Model file for the job. Use its own axes, mm. A direction names the side the tool comes from. Give positions to 0.01 mm unless a question says otherwise; leave off trailing zeros. Write each loop counter-clockwise with the first axis right and the second up, starting at its lowest first coordinate (ties: lowest second). Pieces come first, ordered by that corner, then holes. Notation, with made-up numbers: (-10.5, 86) - (35.5, 86) arc R5 cw to (35.5, 91) - close; hole circle Ø9 at (75.25, 42.5). An arc over 180 degrees is marked (long way). Use CSV: the item, a comma, the result in double quotes.
from build123d import *

# Parameters (mm, degrees)
SKETCH1_W           = 609.6
SKETCH1_H           = 304.8
SKETCH1_W_2         = 93
SKETCH1_H_2         = 93
BOSS_EXTRUDE1_DEPTH = 15.24
SKETCH2_W           = 609.6
SKETCH2_H           = 304.8
BOSS_EXTRUDE2_DEPTH = 3.175
SKETCH3_W           = 609.6
SKETCH3_H           = 304.8
SKETCH3_W_2         = 603.25
SKETCH3_H_2         = 254
BOSS_EXTRUDE3_DEPTH = 30.48
SKETCH4_OUTSIDE_W   = 748.262
SKETCH4_OUTSIDE_H   = 443.462
SKETCH4_OUTSIDE_W_2 = 609.6
SKETCH4_OUTSIDE_H_2 = 260.35
CUT_EXTRUDE1_DEPTH  = 45.72
SKETCH5_R           = 3.4925
CUT_EXTRUDE2_DEPTH  = 344.830071983
SKETCH6_W           = 327.140785269
SKETCH6_H           = 256.091806272
TEMPORARY_CUT_DEPTH = 430.914472374
SKETCH7_W           = 260.35
SKETCH7_H           = 48.895
BOSS_EXTRUDE4_DEPTH = 3.175


with BuildPart() as part:
    # Sketch1 → Boss-Extrude1 (new body)
    with BuildSketch(Plane(origin=(0, 0, 0), x_dir=(1, 0, 0), z_dir=(0, 1, 0))):
        Rectangle(SKETCH1_W, SKETCH1_H)
        with Locations((-48.0875, 29.7)):
            Rectangle(SKETCH1_W_2, SKETCH1_H_2, mode=Mode.SUBTRACT)
        with Locations((-144.2625, 29.7)):
            Rectangle(SKETCH1_W_2, SKETCH1_H_2, mode=Mode.SUBTRACT)
        with Locations((-144.2625, -66.475)):
            Rectangle(SKETCH1_W_2, SKETCH1_H_2, mode=Mode.SUBTRACT)
        with Locations((-48.0875, -66.475)):
            Rectangle(SKETCH1_W_2, SKETCH1_H_2, mode=Mode.SUBTRACT)
        with Locations((-240.4375, 29.7)):
            Rectangle(SKETCH1_W_2, SKETCH1_H_2, mode=Mode.SUBTRACT)
        with Locations((-240.4375, -66.475)):
            Rectangle(SKETCH1_W_2, SKETCH1_H_2, mode=Mode.SUBTRACT)
        with Locations((48.0875, 29.7)):
            Rectangle(SKETCH1_W_2, SKETCH1_H_2, mode=Mode.SUBTRACT)
        with Locations((48.0875, -66.475)):
            Rectangle(SKETCH1_W_2, SKETCH1_H_2, mode=Mode.SUBTRACT)
        with Locations((144.2625, 29.7)):
            Rectangle(SKETCH1_W_2, SKETCH1_H_2, mode=Mode.SUBTRACT)
        with Locations((144.2625, -66.475)):
            Rectangle(SKETCH1_W_2, SKETCH1_H_2, mode=Mode.SUBTRACT)
        with Locations((240.4375, 29.7)):
            Rectangle(SKETCH1_W_2, SKETCH1_H_2, mode=Mode.SUBTRACT)
        with Locations((240.4375, -66.475)):
            Rectangle(SKETCH1_W_2, SKETCH1_H_2, mode=Mode.SUBTRACT)
    extrude(amount=BOSS_EXTRUDE1_DEPTH)

    # Sketch2 → Boss-Extrude2 (add)
    with BuildSketch(Plane(origin=(0, 0, 0), x_dir=(-1, 0, 0), z_dir=(0, -1, 0))):
        Rectangle(SKETCH2_W, SKETCH2_H)
    extrude(amount=BOSS_EXTRUDE2_DEPTH)

    # Sketch3 → Boss-Extrude3 (add)
    with BuildSketch(Plane(origin=(0, 15.24, 0), x_dir=(1, 0, 0), z_dir=(0, 1, 0))):
        Rectangle(SKETCH3_W, SKETCH3_H)
        Rectangle(SKETCH3_W_2, SKETCH3_H_2, mode=Mode.SUBTRACT)
    extrude(amount=BOSS_EXTRUDE3_DEPTH)

    # Sketch4 outside → Cut-Extrude1 (cut)
    with BuildSketch(Plane(origin=(0, 45.72, 0), x_dir=(1, 0, 0), z_dir=(0, 1, 0))):
        Rectangle(SKETCH4_OUTSIDE_W, SKETCH4_OUTSIDE_H)
        Rectangle(SKETCH4_OUTSIDE_W_2, SKETCH4_OUTSIDE_H_2, mode=Mode.SUBTRACT)
    extrude(amount=-CUT_EXTRUDE1_DEPTH, mode=Mode.SUBTRACT)

    # Sketch5 → Cut-Extrude2 (cut, through all)
    with BuildSketch(Plane(origin=(0, 0, 0), x_dir=(1, 0, 0), z_dir=(0, 1, 0))):
        with Locations(Location((-292.1, -139.7, 0), (0, 0, 270))):
            Circle(SKETCH5_R)
        with Locations(Location((-266.7, -139.7, 0), (0, 0, 270))):
            Circle(SKETCH5_R)
        with Locations(Location((-241.3, -139.7, 0), (0, 0, 270))):
            Circle(SKETCH5_R)
        with Locations(Location((-215.9, -139.7, 0), (0, 0, 270))):
            Circle(SKETCH5_R)
        with Locations(Location((-190.5, -139.7, 0), (0, 0, 270))):
            Circle(SKETCH5_R)
        with Locations(Location((-165.1, -139.7, 0), (0, 0, 270))):
            Circle(SKETCH5_R)
        with Locations(Location((-139.7, -139.7, 0), (0, 0, 270))):
            Circle(SKETCH5_R)
        with Locations(Location((-114.3, -139.7, 0), (0, 0, 270))):
            Circle(SKETCH5_R)
        with Locations(Location((-88.9, -139.7, 0), (0, 0, 270))):
            Circle(SKETCH5_R)
        with Locations(Location((-63.5, -139.7, 0), (0, 0, 270))):
            Circle(SKETCH5_R)
        with Locations(Location((-38.1, -139.7, 0), (0, 0, 270))):
            Circle(SKETCH5_R)
        with Locations(Location((-12.7, -139.7, 0), (0, 0, 270))):
            Circle(SKETCH5_R)
        with Locations(Location((12.7, 139.7, 0), (0, 0, 270))):
            Circle(SKETCH5_R)
        with Locations(Location((38.1, 139.7, 0), (0, 0, 270))):
            Circle(SKETCH5_R)
        with Locations(Location((63.5, 139.7, 0), (0, 0, 270))):
            Circle(SKETCH5_R)
        with Locations(Location((88.9, 139.7, 0), (0, 0, 270))):
            Circle(SKETCH5_R)
        with Locations(Location((114.3, 139.7, 0), (0, 0, 270))):
            Circle(SKETCH5_R)
        with Locations(Location((139.7, 139.7, 0), (0, 0, 270))):
            Circle(SKETCH5_R)
        with Locations(Location((165.1, 139.7, 0), (0, 0, 270))):
            Circle(SKETCH5_R)
        with Locations(Location((190.5, 139.7, 0), (0, 0, 270))):
            Circle(SKETCH5_R)
        with Locations(Location((215.9, 139.7, 0), (0, 0, 270))):
            Circle(SKETCH5_R)
        with Locations(Location((241.3, 139.7, 0), (0, 0, 270))):
            Circle(SKETCH5_R)
        with Locations(Location((-292.1, 139.7, 0), (0, 0, 270))):
            Circle(SKETCH5_R)
        with Locations(Location((-266.7, 139.7, 0), (0, 0, 270))):
            Circle(SKETCH5_R)
        with Locations(Location((-241.3, 139.7, 0), (0, 0, 270))):
            Circle(SKETCH5_R)
        with Locations(Location((-215.9, 139.7, 0), (0, 0, 270))):
            Circle(SKETCH5_R)
        with Locations(Location((-190.5, 139.7, 0), (0, 0, 270))):
            Circle(SKETCH5_R)
        with Locations(Location((-165.1, 139.7, 0), (0, 0, 270))):
            Circle(SKETCH5_R)
        with Locations(Location((-139.7, 139.7, 0), (0, 0, 270))):
            Circle(SKETCH5_R)
        with Locations(Location((-114.3, 139.7, 0), (0, 0, 270))):
            Circle(SKETCH5_R)
        with Locations(Location((-88.9, 139.7, 0), (0, 0, 270))):
            Circle(SKETCH5_R)
        with Locations(Location((-63.5, 139.7, 0), (0, 0, 270))):
            Circle(SKETCH5_R)
        with Locations(Location((-38.1, 139.7, 0), (0, 0, 270))):
            Circle(SKETCH5_R)
        with Locations(Location((-12.7, 139.7, 0), (0, 0, 270))):
            Circle(SKETCH5_R)
        with Locations(Location((266.7, 139.7, 0), (0, 0, 270))):
            Circle(SKETCH5_R)
        with Locations(Location((292.1, 139.7, 0), (0, 0, 270))):
            Circle(SKETCH5_R)
        with Locations(Location((12.7, -139.7, 0), (0, 0, 270))):
            Circle(SKETCH5_R)
        with Locations(Location((38.1, -139.7, 0), (0, 0, 270))):
            Circle(SKETCH5_R)
        with Locations(Location((63.5, -139.7, 0), (0, 0, 270))):
            Circle(SKETCH5_R)
        with Locations(Location((88.9, -139.7, 0), (0, 0, 270))):
            Circle(SKETCH5_R)
        with Locations(Location((114.3, -139.7, 0), (0, 0, 270))):
            Circle(SKETCH5_R)
        with Locations(Location((139.7, -139.7, 0), (0, 0, 270))):
            Circle(SKETCH5_R)
        with Locations(Location((165.1, -139.7, 0), (0, 0, 270))):
            Circle(SKETCH5_R)
        with Locations(Location((190.5, -139.7, 0), (0, 0, 270))):
            Circle(SKETCH5_R)
        with Locations(Location((215.9, -139.7, 0), (0, 0, 270))):
            Circle(SKETCH5_R)
        with Locations(Location((241.3, -139.7, 0), (0, 0, 270))):
            Circle(SKETCH5_R)
        with Locations(Location((266.7, -139.7, 0), (0, 0, 270))):
            Circle(SKETCH5_R)
        with Locations(Location((292.1, -139.7, 0), (0, 0, 270))):
            Circle(SKETCH5_R)
    extrude(amount=-CUT_EXTRUDE2_DEPTH, mode=Mode.SUBTRACT)

    # Sketch6 → Temporary_Cut (cut, through all)
    with BuildSketch(Plane(origin=(-94.5875, 0, 0), x_dir=(0, 0, -1), z_dir=(1, 0, 0))):
        with Locations((-7.828616148, 44.910513642)):
            Rectangle(SKETCH6_W, SKETCH6_H)
    extrude(amount=TEMPORARY_CUT_DEPTH, mode=Mode.SUBTRACT)

    # Sketch7 → Boss-Extrude4 (add)
    with BuildSketch(Plane(origin=(-94.5875, 0, 0), x_dir=(0, 0, -1), z_dir=(1, 0, 0))):
        with Locations((0, 21.2725)):
            Rectangle(SKETCH7_W, SKETCH7_H)
    extrude(amount=BOSS_EXTRUDE4_DEPTH)


solid = part.part
(1) Wall check: probe 1 along Z at (x, y) = (-210, 10) (3 decimals); probe 2 along Z at (x, y) = (-190.5, -0.9); probe 3 along Z at (x, y) = (-279, 41) (3 decimals). Give the ranges that are in metal, low to high. Write a range as [from, to].
Checked values:
probe 1,"z = [-130.175, -76.2], [16.8, 19.975], [112.975, 130.175]"
probe 2,"z = [-152.4, -143.19], [-136.21, 136.21], [143.19, 152.4]"
probe 3,"z = [-130.175, -127], [127, 130.175]"
(2) Saw through at A-A, the plane x = -292.1. List the corners of the cut face in (y, z) (1 decimal).
Checked values:
outline,"(-3.2, -152.4) - (0, -152.4) - (0, -143.2) - (-3.2, -143.2) - close; (-3.2, -136.2) - (0, -136.2) - (0, -130.2) - (45.7, -130.2) - (45.7, -127) - (15.2, -127) - (15.2, 127) - (45.7, 127) - (45.7, 130.2) - (0, 130.2) - (0, 136.2) - (-3.2, 136.2) - close; (-3.2, 143.2) - (0, 143.2) - (0, 152.4) - (-3.2, 152.4) - close"
(3) Saw through at B-B, the plane y = 10.5. List the corners of the cut face in (x, z) (1 decimal).
Checked values:
outline,"(-304.8, -130.2) - (-91.4, -130.2) - (-91.4, 130.2) - (-304.8, 130.2) - close; hole (-286.9, -76.2) - (-193.9, -76.2) - (-193.9, 16.8) - (-286.9, 16.8) - close; hole (-286.9, 20) - (-193.9, 20) - (-193.9, 113) - (-286.9, 113) - close; hole (-190.8, -76.2) - (-97.8, -76.2) - (-97.8, 16.8) - (-190.8, 16.8) - close; hole (-190.8, 20) - (-97.8, 20) - (-97.8, 113) - (-190.8, 113) - close"
(4) Saw through at D-D, the plane x = -114.3. List the corners of the cut face in (y, z) (1 decimal), then the cut area to 3 significant figures.
Checked values:
outline,"(-3.2, -152.4) - (0, -152.4) - (0, -143.2) - (-3.2, -143.2) - close; (-3.2, -136.2) - (0, -136.2) - (0, -130.2) - (45.7, -130.2) - (45.7, -127) - (15.2, -127) - (15.2, -76.2) - (0, -76.2) - (0, 16.8) - (15.2, 16.8) - (15.2, 20) - (0, 20) - (0, 113) - (15.2, 113) - (15.2, 127) - (45.7, 127) - (45.7, 130.2) - (0, 130.2) - (0, 136.2) - (-3.2, 136.2) - close; (-3.2, 143.2) - (0, 143.2) - (0, 152.4) - (-3.2, 152.4) - close"
area,"2,250 mm^2"
(5) 3-axis set-ups, long thin cutter, end or side, ignore diameter. For faces 5 (the face through (-193.938, 8, -29)), 6 (the face through (-288.637, -1.565, 139.245)): which of +Z, -Z, +X, -X, +Y, -Y reach the whole face in a straight line?
Checked values:
face 5,"+Y"
face 6,"+Y, -Y"
(6) Pull direction X, two halves, no side cores. Call faces 1 (the face through (-304.8, 21, 2)), 2 (the face through (-244.4, -1.57, -138.09)), 3 (the face through (-200, 21, 130.175)), 4 (the face through (-190.762, 8, -29)): released by +X, released by -X, zero draft, split by the parting line, or undercut.
Checked values:
face 1,"released by -X"
face 2,"undercut"
face 3,"zero draft"
face 4,"undercut"
(7) Saw through at C-C, the plane z = 6. List the corners of the cut face in (x, y) (1 decimal), then the cut area to 3 significant figures.
Checked values:
outline,"(-304.8, -3.2) - (-91.4, -3.2) - (-91.4, 45.7) - (-94.6, 45.7) - (-94.6, 15.2) - (-97.8, 15.2) - (-97.8, 0) - (-190.8, 0) - (-190.8, 15.2) - (-193.9, 15.2) - (-193.9, 0) - (-286.9, 0) - (-286.9, 15.2) - (-301.6, 15.2) - (-301.6, 45.7) - (-304.8, 45.7) - close"
area,"1,290 mm^2"
(8) Flat gauge pins, fed straight in: P1, Ø10, axis at x = -119.5, y = 40, coming from the -Z side (3 decimals); P2, Ø1, axis at x = -218.5, z = 59.5, coming from the +Y side; P3, Ø24.5, axis at x = -244.5, y = 27.5, coming from the +Z side (3 decimals). Where does each tip first touch, or does it go through?
Checked values:
P1,"stops at z = -130.175"
P2,"stops at y = 0"
P3,"stops at z = 130.175"
